Geometry: final body of the model. Coordinates: model frame, mm. Give positions to 0.01 mm unless a question says otherwise; leave off trailing zeros. Write each loop counter-clockwise with the first axis right and the second up, starting at its lowest first coordinate (ties: lowest second). Pieces come first, ordered by that corner, then holes. Notation, with made-up numbers: (82, -32) -> (102, -32) arc R23 ccw to (102, -24) -> close; hole circle Ø1 at (2.5, 17). An arc over 180 degrees is marked (long way). Answer in a Markdown table with one row per item. Add a question column.
Item 1: Section query C-C on z = 2.4. Output: boundary loops of the cut face in (x, y).
Item 2: Section query A-A on x = 0. Output: boundary loops of the cut face in (y, z), plus the area to 3 significant figures.
Item 3: Draft query along X for faces 1 (the cylindrical face through (-5.58, -25.14, 2.52)), 2 (the cylindrical face through (-4.88, 37.18, 2.46)), 3 (the flat face through (8, 26, 0)). Return one class per face: +X half, -X half, draft (parallel to the pull), parting line (faces both ways), or undercut.
Item 4: First-contact query: P1, Ø2, axis at x = -10, z = 2, coming from the -Y side; P2, Ø3, axis at x = -24, z = 1.5, coming from the +Y side. Flat tips, straight axial feed; report the tip coordinate or a pass-through.
Item 5: Material intervals for probe 1 along Y at (x, z) = (0, 2.4); probe 2 along X at (y, z) = (4, 0.75); probe 3 along Y at (x, z) = (-23.5, 1.25), sorted ascending. Write a range as from..to.
Item 6: Section query D-D on y = 29. Output: boundary loops of the cut face in (x, z).
```python
from build123d import *

# Parameters (mm, degrees)
GUARD_BASE_R     = 37.5
GUARD_DEPTH      = 5
AXLE_HOLE_BASE_R = 25.75
AXLE_HOLE_DEPTH  = 6


with BuildPart() as part:
    # Guard base → Guard (new body)
    with BuildSketch(Plane.XY):
        Circle(GUARD_BASE_R)
    extrude(amount=GUARD_DEPTH)

    # Axle hole base → Axle hole (cut, through all)
    with BuildSketch(Plane.XY.offset(5)):
        Circle(AXLE_HOLE_BASE_R)
    extrude(amount=-AXLE_HOLE_DEPTH, mode=Mode.SUBTRACT)

    # Mate ring room base → Mate ring room (revolve, cut)
    with BuildSketch(Plane(origin=(0, 0, 0), x_dir=(1, 0, 0), z_dir=(0, 1, 0))):
        Polygon((25.75, -5), (26.5, -5), (25.75, -4.25), align=None)
        Polygon((25.75, 0), (26.5, 0), (25.75, -0.75), align=None)
    revolve(axis=Axis((0, 0, 0), (0, 0, -1)), mode=Mode.SUBTRACT)


solid = part.part
```
Findings below:
| question | item | result |
|---|---|---|
| 1 | outline | circle Ø75 at (0, 0); hole circle Ø51.5 at (0, 0) |
| 2 | outline | (-37.5, 0) -> (-26.5, 0) -> (-25.75, 0.75) -> (-25.75, 4.25) -> (-26.5, 5) -> (-37.5, 5) -> close; (25.75, 0.75) -> (26.5, 0) -> (37.5, 0) -> (37.5, 5) -> (26.5, 5) -> (25.75, 4.25) -> close |
| 2 | area | 116 mm^2 |
| 3 | face 1 | undercut |
| 3 | face 2 | parting line |
| 3 | face 3 | draft |
| 4 | P1 | stops at y = -36.4 |
| 4 | P2 | stops at y = 30 |
| 5 | probe 1 | y = -37.5..-25.75, 25.75..37.5 |
| 5 | probe 2 | x = -37.29..-25.44, 25.44..37.29 |
| 5 | probe 3 | y = -29.22..-10.53, 10.53..29.22 |
| 6 | outline | (-23.77, 0) -> (23.77, 0) -> (23.77, 5) -> (-23.77, 5) -> close |
